Check sheet for the modelled part. Datum: model origin and axes. Units: mm. A direction names the side the tool comes from. Coordinates: 2 decimals unless noted, no trailing zeros. Loops run counter-clockwise (first coordinate to the right, second up) from the corner with the lowest first, then second, coordinate; pieces in that order, holes last. Notation, with made-up numbers: M 3.5,73.5 L 43.5,73.5 A18 cw 43.5,90.5 Z; hole C -23.5,14 d5. An arc over 180 degrees is marked long. Return JSON: item names as keys, results as strings.
from build123d import *

# Parameters (mm, degrees)
SKETCH_1_R      = 60
EXTRUDE_1_DEPTH = 5
SKETCH_2_R      = 60
SKETCH_2_R_2    = 57
EXTRUDE_2_DEPTH = 3
EXTRUDE_3_DEPTH = 3


with BuildPart() as part:
    # 草图1 → 凸台-拉伸1 (new body)
    with BuildSketch(Plane.XY):
        Circle(SKETCH_1_R)
        with BuildLine():
            Line((-43.97114317, -13.839745962), (-33.97114317, -31.160254038))
            ThreePointArc((-33.97114317, -31.160254038), (-35.801270189, -37.990381057), (-42.631397208, -36.160254038))
            Line((-42.631397208, -36.160254038), (-52.631397208, -18.839745962))
            ThreePointArc((-52.631397208, -18.839745962), (-50.801270189, -12.009618943), (-43.97114317, -13.839745962))
        make_face(mode=Mode.SUBTRACT)
        with BuildLine():
            Line((43.97114317, -13.839745962), (33.97114317, -31.160254038))
            ThreePointArc((33.97114317, -31.160254038), (35.801270189, -37.990381057), (42.631397208, -36.160254038))
            Line((42.631397208, -36.160254038), (52.631397208, -18.839745962))
            ThreePointArc((52.631397208, -18.839745962), (50.801270189, -12.009618943), (43.97114317, -13.839745962))
        make_face(mode=Mode.SUBTRACT)
        with BuildLine():
            Line((10, 45), (-10, 45))
            ThreePointArc((-10, 45), (-15, 50), (-10, 55))
            Line((-10, 55), (10, 55))
            ThreePointArc((10, 55), (15, 50), (10, 45))
        make_face(mode=Mode.SUBTRACT)
    extrude(amount=EXTRUDE_1_DEPTH)

    # 草图2 → 凸台-拉伸2 (add)
    with BuildSketch(Plane.XY.offset(5)):
        Circle(SKETCH_2_R)
        Circle(SKETCH_2_R_2, mode=Mode.SUBTRACT)
    extrude(amount=EXTRUDE_2_DEPTH)

    # 草图3 → 凸台-拉伸3 (add)
    with BuildSketch(Plane.XY.offset(5)):
        with BuildLine():
            Line((48.333051801, 30.214501545), (0, 2.309401077))
            Line((0, 2.309401077), (-48.333051801, 30.214501545))
            ThreePointArc((-48.333051801, 30.214501545), (-49.363448016, 28.5), (-50.333051801, 26.75039993))
            Line((-50.333051801, 26.75039993), (-2, -1.154700538))
            Line((-2, -1.154700538), (-2, -56.964901475))
            ThreePointArc((-2, -56.964901475), (0, -57), (2, -56.964901475))
            Line((2, -56.964901475), (2, -1.154700538))
            Line((2, -1.154700538), (50.333051801, 26.75039993))
            ThreePointArc((50.333051801, 26.75039993), (49.363448016, 28.5), (48.333051801, 30.214501545))
        make_face()
    extrude(amount=EXTRUDE_3_DEPTH)


solid = part.part
1) Section check A-A on y = 50. Record the cut outline in (x, z).
Answers:
{"outline": "M -33.17,0 L -15,0 L -15,5 L -27.37,5 L -27.37,8 L -33.17,8 Z; M 15,0 L 33.17,0 L 33.17,8 L 27.37,8 L 27.37,5 L 15,5 Z"}
2) Go/stop test with flat-tipped pins: pin 1 Ø4 at (x, z) = (-9.5, 2) entering from +Y; pin 2 Ø3 at (x, z) = (-42.5, 5) entering from +Y; pin 3 Ø2.5 at (y, z) = (-38.5, 6) entering from +X. Record where each tip stops, or that it passes through.
Answers:
{"pin 1": "y = 59.53", "pin 2": "y = 43.81", "pin 3": "x = 47.04"}
3) Section check B-B on y = -20.5. Record the cut outline in (x, z).
Answers:
{"outline": "M -56.39,0 L -51.67,0 L -51.67,5 L -53.19,5 L -53.19,8 L -56.39,8 Z; M -40.13,0 L 40.13,0 L 40.13,5 L 2,5 L 2,8 L -2,8 L -2,5 L -40.13,5 Z; M 51.67,0 L 56.39,0 L 56.39,8 L 53.19,8 L 53.19,5 L 51.67,5 Z"}
4) Section check C-C on x = -24. Record the cut outline in (y, z).
Answers:
{"outline": "M -54.99,0 L 54.99,0 L 54.99,8 L 51.7,8 L 51.7,5 L 16.17,5 L 16.17,8 L 11.55,8 L 11.55,5 L -51.7,5 L -51.7,8 L -54.99,8 Z"}
5) Scan lines: line 1 along X through (y, z) = (-37.5, 4.75); line 2 along X through (y, z) = (-26.5, 2); line 3 along Y through (x, z) = (-9, 7.5). Record each from-to range of solid material in increasing order. Write a range as [from, to].
Answers:
{"line 1": "[-46.84, -41.5], [-35.1, 35.1], [41.5, 46.84]", "line 2": "[-53.83, -48.21], [-36.66, 36.66], [48.21, 53.83]", "line 3": "[-59.32, -56.28], [2.89, 7.51], [56.28, 59.32]"}
6) Set-up check for faces 1 (the face through (15, 50, 2)), 2 (the face through (-1, 1, 0)), 3 (the face through (25.828, 12.603, 6.479)): record each of +Z, -Z, +X, -X, +Y, -Y from which the full face is reachable in a straight line by a thin tool's end or side.
Answers:
{"face 1": "+Z, -Z", "face 2": "-Z, +X, -X, +Y, -Y", "face 3": "+Z"}
7) Draft check along X on faces 4 (the face through (0, 0, 8)), 5 (the face through (-2, -29, 6)). Enter one of: +X half, -X half, draft (parallel to the pull), parting line (faces both ways), or undercut.
Answers:
{"face 4": "draft", "face 5": "undercut"}
